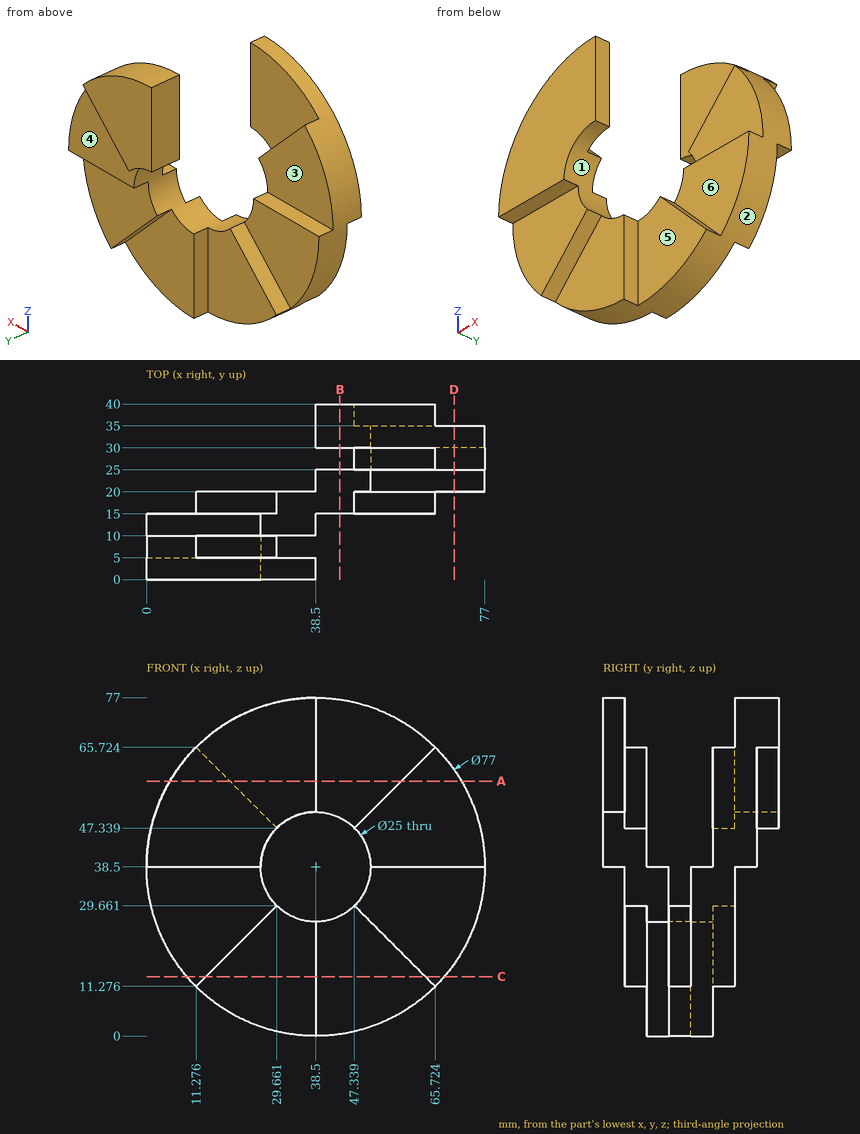
Verification items for this drawing (mm, ordinates from the low corner). A direction names the side the tool comes from. Give positions to 0.01 mm unless a question says otherwise; leave off trailing zeros. Write each loop counter-clockwise with the first axis right and the second up, starting at its lowest first coordinate (ties: lowest second). Pieces come first, ordered by that corner, then holes.
1) Thickness scan on line 1 (Y direction, x = 32.5, z = 53); line 2 (Y direction, x = 29.5, z = 28); line 3 (Z direction, x = 43, y = 35.5) (1 decimal). Record the ranges inside material, lowest first.
Values follow:
line 1: y = 0 to 5
line 2: y = 10 to 20
line 3: z = 50.2 to 76.7
2) Cross-section at B-B (x = 44). Record the boundary of the cut face in (y, z) (1 decimal).
Values follow:
outline: (15, 0.4) - (25, 0.4) - (25, 27.3) - (15, 27.3) - close; (30, 49.7) - (40, 49.7) - (40, 76.6) - (30, 76.6) - close
3) Go/stop test with flat-tipped pins: pin 1 Ø5.5 at (y, z) = (12, 8.5) entering from +X; pin 2 Ø10 at (y, z) = (10, 68) entering from -X; pin 3 Ø13.5 at (x, z) = (45.5, 11) entering from -Y. Record where each tip stops, or that it passes through.
Values follow:
pin 1: stops at x = 38.5
pin 2: stops at x = 8.8
pin 3: stops at y = 15
4) Cross-section at C-C (z = 13.5). Record the boundary of the cut face in (x, y).
Values follow:
outline: (9.22, 5) - (13.5, 5) - (13.5, 10) - (38.5, 10) - (38.5, 15) - (63.5, 15) - (63.5, 20) - (67.78, 20) - (67.78, 30) - (63.5, 30) - (63.5, 25) - (38.5, 25) - (38.5, 20) - (13.5, 20) - (13.5, 15) - (9.22, 15) - close
5) Cross-section at D-D (x = 70). Record the boundary of the cut face in (y, z).
Values follow:
outline: (20, 16.36) - (30, 16.36) - (30, 38.5) - (35, 38.5) - (35, 60.64) - (25, 60.64) - (25, 38.5) - (20, 38.5) - close
6) Cross-section at A-A (z = 58). Record the boundary of the cut face in (x, y).
Values follow:
outline: (5.3, 0) - (38.5, 0) - (38.5, 5) - (19, 5) - (19, 10) - (5.3, 10) - close; (38.5, 30) - (58, 30) - (58, 25) - (71.7, 25) - (71.7, 35) - (58, 35) - (58, 40) - (38.5, 40) - close
7) Set-up check for the marked faces 4, 5 and 6: record each of +Z, -Z, +X, -X, +Y, -Y from which the full face is reachable in a straight line by a thin tool's end or side.
Values follow:
face 4: -Z, +X, +Y
face 5: +Z, -Z, +X, -Y
face 6: +Z, +X, -Y
8) Release check for a two-part mould opening along Z. For the marked faces 1, 2 and 3 record: released by +Z, released by -Z, zero draft, split by the parting line, or undercut.
Values follow:
face 1: undercut
face 2: split by the parting line
face 3: zero draft
